```python
from build123d import *

# Parameters (mm, degrees)
TAP_DRILL_FOR_M12X1_25_TAP1_D     = 12
TAP_DRILL_FOR_M12X1_25_TAP1_DEPTH = 7.394836286
TAP_DRILL_FOR_M12X1_25_TAP1_TIP   = 3.605163714
SKETCH5_R                         = 4
CUT_EXTRUDE1_DEPTH                = 40.525308348
CUT_EXTRUDE2_DEPTH                = 39.105117767
CUT_EXTRUDE2_DEPTH_BACK           = 39.105117767
SKETCH6_R                         = 2


with BuildPart() as part:
    # Sketch1 → Revolve1 (revolve)
    with BuildSketch(Plane.XY, mode=Mode.PRIVATE) as revolve1_sk:
        Polygon((0, 7.25), (0, -7.25), (12, -7.25), (12, 2.75), (26, 2.75), (26, 6.25), (15, 6.25), (15, 7.25), align=None)
    revolve(revolve1_sk.sketch.rotate(Axis((0, 11.233516484, 0), (0, -1, 0)), 90), axis=Axis((0, 11.233516484, 0), (0, -1, 0)))

    # Tap Drill for M12x1.25 Tap1
    with Locations(Plane(origin=(0, -7.25, 0), x_dir=(-1, 0, 0), z_dir=(0, -1, 0))):
        with Locations((0, 0)):
            Hole(TAP_DRILL_FOR_M12X1_25_TAP1_D / 2, depth=TAP_DRILL_FOR_M12X1_25_TAP1_DEPTH)
            with Locations((0, 0, -(TAP_DRILL_FOR_M12X1_25_TAP1_DEPTH + TAP_DRILL_FOR_M12X1_25_TAP1_TIP / 2))):  # 118° drill point
                Cone(0, TAP_DRILL_FOR_M12X1_25_TAP1_D / 2, TAP_DRILL_FOR_M12X1_25_TAP1_TIP, mode=Mode.SUBTRACT)

    # Sketch5 → Cut-Extrude1 (cut, through all)
    with BuildSketch(Plane(origin=(0, 7.25, 0), x_dir=(1, 0, 0), z_dir=(0, 1, 0))):
        with Locations(Location((0, 0, 0), (0, 0, 270))):
            Circle(SKETCH5_R)
    extrude(amount=-CUT_EXTRUDE1_DEPTH, mode=Mode.SUBTRACT)

    # Sketch6 → Cut-Extrude2 (cut, two sides: drawn at the far end of the back side and taken through both)
    with BuildSketch(Plane.XZ.offset(-2.75).offset(-CUT_EXTRUDE2_DEPTH_BACK)):
        with Locations(Location((-18.619546181, 10.75, 0), (0, 0, 270))):
            Circle(SKETCH6_R)
        with Locations(Location((0, 21.5, 0), (0, 0, 270))):
            Circle(SKETCH6_R)
        with Locations(Location((18.619546181, 10.75, 0), (0, 0, 270))):
            Circle(SKETCH6_R)
        with Locations(Location((18.619546181, -10.75, 0), (0, 0, 270))):
            Circle(SKETCH6_R)
        with Locations(Location((0, -21.5, 0), (0, 0, 270))):
            Circle(SKETCH6_R)
        with Locations(Location((-18.619546181, -10.75, 0), (0, 0, 270))):
            Circle(SKETCH6_R)
    extrude(amount=CUT_EXTRUDE2_DEPTH + CUT_EXTRUDE2_DEPTH_BACK, mode=Mode.SUBTRACT)


solid = part.part
```
Design review of the part built by this model. Coordinates are the model's own, in mm. A direction names the side the tool comes from. Give positions to 0.01 mm unless a question says otherwise; leave off trailing zeros. Loops run counter-clockwise (first coordinate to the right, second up) from the corner with the lowest first, then second, coordinate; pieces in that order, holes last. Notation, with made-up numbers: (69.25, 88) -> (104.25, 88) arc R10 ccw to (104.25, 102) -> close; hole circle Ø11 at (-5.5, -10.5). An arc over 180 degrees is marked (long way). Write each question's results on one line, items separated by ' | '.
Q1. The part is to be moulded in two halves that separate along X. For faces 4 (the face through (-1.2, 4.5, 23.1)), 5 (the face through (3, 7.25, 3)), 6 (the face through (-12.65, 6.76, 8.06)), say which applies: +X half, -X half, draft (parallel to the pull), parting line (faces both ways), or undercut.
Reply:
face 4: undercut | face 5: draft | face 6: parting line
Q2. Take a section at C-C, the plane y = 5.25. Write out the cut boundary in (x, z).
Reply:
outline: circle Ø52 at (0, 0); hole circle Ø4 at (-18.62, -10.75); hole circle Ø4 at (-18.62, 10.75); hole circle Ø8 at (0, 0); hole circle Ø4 at (0, -21.5); hole circle Ø4 at (0, 21.5); hole circle Ø4 at (18.62, -10.75); hole circle Ø4 at (18.62, 10.75)
Q3. Wall thickness on L1, parallel to X at y = 5.3, z = -10.75; L2, parallel to Z at x = -1.5, y = 4; L3, parallel to Y at x = -19, z = 17.5: over which ranges is each line inside the solid? List them lowest first.
Reply:
L1: x = -23.67 to -20.62, -16.62 to 16.62, 20.62 to 23.67 | L2: z = -25.96 to -22.82, -20.18 to -3.71, 3.71 to 20.18, 22.82 to 25.96 | L3: y = 2.75 to 6.25
Q4. Take a section at D-D, the plane z = -10.75. Write out the cut boundary in (x, y).
Reply:
outline: (-23.67, 2.75) -> (-20.62, 2.75) -> (-20.62, 6.25) -> (-23.67, 6.25) -> close; (-16.62, 2.75) -> (-5.33, 2.75) -> (-5.33, -7.25) -> (5.33, -7.25) -> (5.33, 2.75) -> (16.62, 2.75) -> (16.62, 6.25) -> (10.46, 6.25) -> (10.46, 7.25) -> (-10.46, 7.25) -> (-10.46, 6.25) -> (-16.62, 6.25) -> close; (20.62, 2.75) -> (23.67, 2.75) -> (23.67, 6.25) -> (20.62, 6.25) -> close
Q5. Take a section at B-B, the plane z = 21.5. Write out the cut boundary in (x, y).
Reply:
outline: (-14.62, 2.75) -> (-2, 2.75) -> (-2, 6.25) -> (-14.62, 6.25) -> close; (2, 2.75) -> (14.62, 2.75) -> (14.62, 6.25) -> (2, 6.25) -> close
Q6. Take a section at A-A, the plane x = 0. Write out the cut boundary in (y, z).
Reply:
outline: (-7.25, -12) -> (2.75, -12) -> (2.75, -19.5) -> (6.25, -19.5) -> (6.25, -15) -> (7.25, -15) -> (7.25, -4) -> (1.35, -4) -> (0.14, -6) -> (-7.25, -6) -> close; (-7.25, 6) -> (0.14, 6) -> (1.35, 4) -> (7.25, 4) -> (7.25, 15) -> (6.25, 15) -> (6.25, 19.5) -> (2.75, 19.5) -> (2.75, 12) -> (-7.25, 12) -> close; (2.75, -26) -> (6.25, -26) -> (6.25, -23.5) -> (2.75, -23.5) -> close; (2.75, 23.5) -> (6.25, 23.5) -> (6.25, 26) -> (2.75, 26) -> close
Q7. Machinability: for faces 1 (the face through (11, 6.25, 11)), 2 (the face through (-6, -4, 0)), 3 (the face through (-19.837, 4.525, 12.337)), which of the approach directions +Z, -Z, +X, -X, +Y, -Y give a long, thin tool a straight path to every point of the face, cutting with its end or side? Answer none if there is none.
Reply:
face 1: +Y | face 2: -Y | face 3: +Y, -Y
Q8. For pin 1 Ø1.5 at (x, y) = (2, 4.5) entering from -Z; pin 2 Ø3.5 at (x, z) = (0, -21.5) entering from -Y; pin 3 Ø3 at (y, z) = (5.5, -4.5) entering from +X; pin 4 Ø9 at (x, z) = (0, 0) entering from +Y, all flat-tipped, find the tip position at first contact; note any pin that passes through.
Reply:
pin 1: stops at z = -25.97 | pin 2: passes through | pin 3: stops at x = 25.83 | pin 4: stops at y = 7.25
